Model file for the job. Use its own axes, mm. Face numbers are marked on the shaded views. A direction names the side the tool comes from. Coordinates: 2 decimals unless noted, no trailing zeros. Write each loop counter-clockwise with the first axis right and the second up, starting at its lowest first coordinate (ties: lowest second). Pieces come first, ordered by that corner, then holes. Notation, with made-up numbers: M -35.5,60.5 L 20.5,60.5 A20 ccw 20.5,93.5 Z; hole C -38,37.25 d10. An arc over 180 degrees is marked long. Answer in a Markdown table with one row per item. Add a question column.
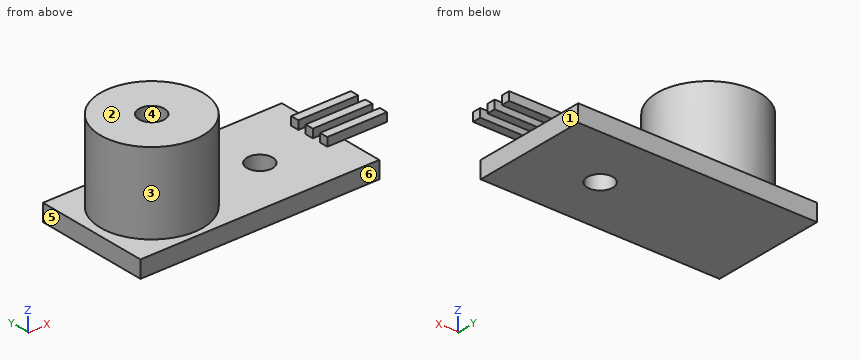
```python
from build123d import *

# Parameters (mm, degrees)
F0_W     = 28
F0_H     = 13.5
F1_DEPTH = 2
F2_R     = 6
F3_DEPTH = 9.5
F4_R     = 1.5
F5_DEPTH = 2
F6_W     = 7
F6_H     = 1
F7_DEPTH = 1
F8_R     = 1.5
F9_DEPTH = 25


with BuildPart() as f1:
    # F0 (on Top) → F1 (new body)
    with BuildSketch(Plane.XY):
        with Locations((14, -6.75)):
            Rectangle(F0_W, F0_H)
    extrude(amount=F1_DEPTH)

    # F2 (on face) → F3 (join)
    with BuildSketch(Plane.XY.offset(2)):
        with Locations((6.98589, -6.804436)):
            Circle(F2_R)
    extrude(amount=F3_DEPTH)

    # F4 (on face) → F5 (cut)
    with BuildSketch(Plane.XY.offset(11.5)):
        with Locations((6.98589, -6.804436)):
            Circle(F4_R)
    extrude(amount=-F5_DEPTH, mode=Mode.SUBTRACT)

    # F6 (on face) → F7 (join)
    with BuildSketch(Plane.XY.offset(2)):
        with Locations((29.494992, -8.169937)):
            Rectangle(F6_W, F6_H)
        with Locations((29.494992, -6.169937)):
            Rectangle(F6_W, F6_H)
        with Locations((29.494992, -4.169937)):
            Rectangle(F6_W, F6_H)
    extrude(amount=F7_DEPTH)

    # F8 (on face) → F9 (cut)
    with BuildSketch(Plane.XY.offset(2)):
        with Locations((19.5, -7)):
            Circle(F8_R)
    extrude(amount=-F9_DEPTH, mode=Mode.SUBTRACT)


solid = f1.part
```
1) Slice it at A-A (x = 19.5). Give the cut face in (y, z), then the cut area to 3 significant figures.
2) Slice it at D-D (x = 13.5). Give the cut face in (y, z).
3) Drill centre lines: probe 1 along Y at (x, z) = (19.5, 0.65); probe 2 along Z at (x, y) = (25.5, -1.75); probe 3 along X at (y, z) = (-4.5, 0.5). Where is each one in solid material? Low to high.
4) Flat gauge pins, fed straight in: pin 1 Ø2 at (x, z) = (12.5, 5) entering from +Y; pin 2 Ø0.8 at (x, z) = (28, 2.5) entering from -Y; pin 3 Ø5 at (y, z) = (-10.5, 5.5) entering from +X. Where does each tip first touch, or does it go through?
5) Which spindle directions (+Z, -Z, +X, -X, +Y, -Y) get a long thin tool onto all of the face, cutting with end or side? Do the marked faces 1 and 2. Say none if no direction does.
6) Slice it at C-C (y = -1.5). Give the cut face in (x, z).
7) Slice it at B-B (y = -8). Give the cut face in (x, z) (3 decimals), then the cut area to 3 significant figures.
8) Two-plate mould, pull along Y, no slides. Class the marked faces 3, 4, 5 and 6: released by +Y, released by -Y, zero draft, split by the parting line, or undercut.
Ans:
| question | item | result |
|---|---|---|
| 1 | outline | M -13.5,0 L -8.5,0 L -8.5,2 L -13.5,2 Z; M -5.5,0 L 0,0 L 0,2 L -5.5,2 Z |
| 1 | area | 21.0 mm2 |
| 2 | outline | M -13.5,0 L 0,0 L 0,2 L -13.5,2 Z |
| 3 | probe 1 | y = -13.5 to -8.5, -5.5 to 0 |
| 3 | probe 2 | z = 0 to 2 |
| 3 | probe 3 | x = 0 to 28 |
| 4 | pin 1 | stops at y = -2.85 |
| 4 | pin 2 | stops at y = -8.67 |
| 4 | pin 3 | stops at x = 12.87 |
| 5 | face 1 | -Z, +X, +Y, -Y |
| 5 | face 2 | +Z, +X, -X, +Y, -Y |
| 6 | outline | M 0,0 L 28,0 L 28,2 L 9.79,2 L 9.79,11.5 L 4.18,11.5 L 4.18,2 L 0,2 Z |
| 7 | outline | M 0,0 L 18.382,0 L 18.382,2 L 12.866,2 L 12.866,11.5 L 7.892,11.5 L 7.892,9.5 L 6.08,9.5 L 6.08,11.5 L 1.106,11.5 L 1.106,2 L 0,2 Z; M 20.618,0 L 28,0 L 28,2 L 32.995,2 L 32.995,3 L 25.995,3 L 25.995,2 L 20.618,2 Z |
| 7 | area | 167 mm2 |
| 8 | face 3 | split by the parting line |
| 8 | face 4 | undercut |
| 8 | face 5 | zero draft |
| 8 | face 6 | released by -Y |
